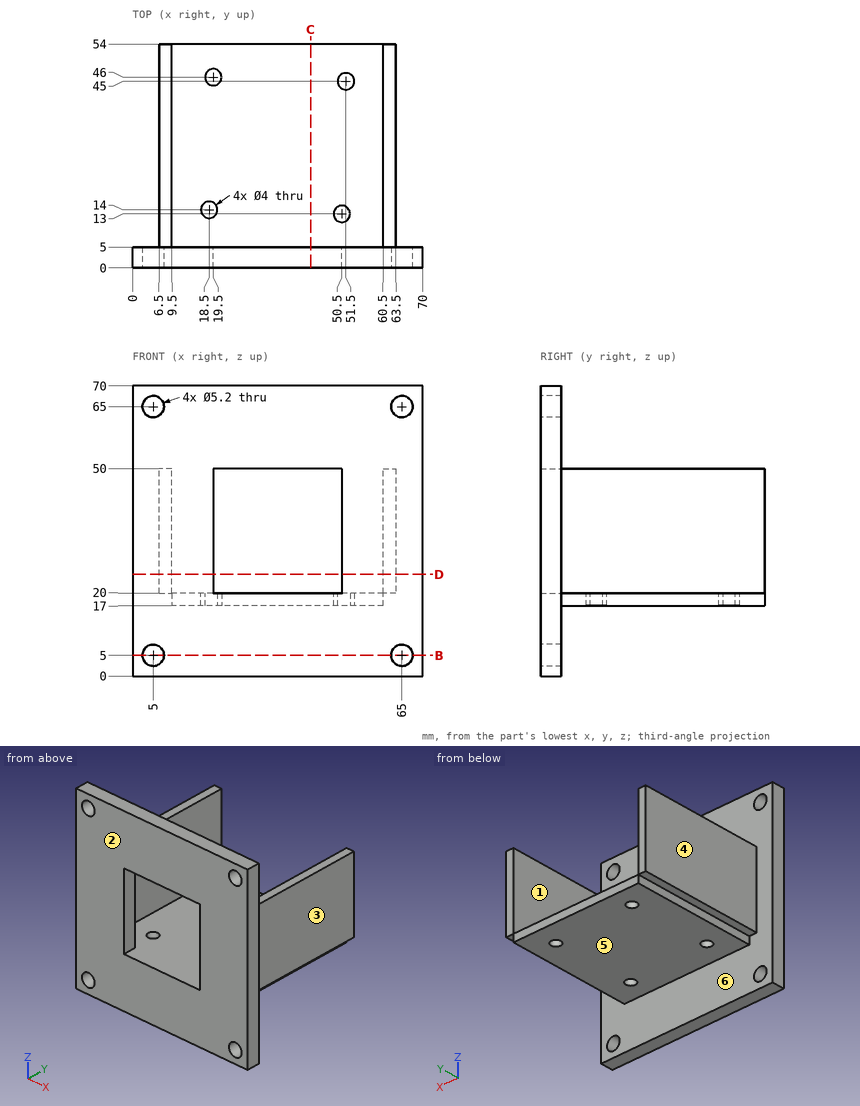
The drawing under review shows one solid part. Ordinate dimensions are in mm from its lowest x, y, z. A direction names the side the tool comes from. Round coordinates to 2 decimals unless told otherwise and drop trailing zeros. Loops run counter-clockwise (first coordinate to the right, second up) from the corner with the lowest first, then second, coordinate; pieces in that order, holes last. Notation, with made-up numbers: (44.25, 80.5) - (84.25, 80.5) arc R13 ccw to (84.25, 102.5) - close; hole circle Ø3 at (30.5, -23.5). An arc over 180 degrees is marked (long way). One line per item, written item: value. Start each with the question number.
1) To check wall thickness, follow L1, parallel to Z at x = 5, y = 1.9; L2, parallel to X at y = 28, z = 22.5; L3, parallel to Z at x = 39, y = 2. State the ranges of each line that lie inside material, in increasing order. Write a range as from..to.
2) Consider section C-C on x = 43. Give the boundary of the cut face in (y, z), then the cut area to 3 significant figures.
3) For the marked faces 1, 2 and 3, list the 3-axis set-ups (+Z, -Z, +X, -X, +Y, -Y) from which the entire face can be reached by the end or side of a thin tool; tool diameter is ignored.
4) Insertion check: pin 1 Ø6 at (x, z) = (58, 18) entering from -Y; pin 2 Ø0.9 at (x, y) = (61.5, 22.5) entering from +Z; pin 3 Ø12 at (y, z) = (41.5, 54) entering from -X; pin 4 Ø2 at (y, z) = (31.5, 28.5) entering from +X. Each pin has a flat end and moves straight along its axis. Give the tip position at first contact, or say it passes through.
5) Consider section D-D on z = 24.5. Give the boundary of the cut face in (x, y).
6) Draft analysis for pull direction X (two halves, no side actions). For the marked faces 4, 5 and 6, state which applies: +X half, -X half, draft (parallel to the pull), parting line (faces both ways), or undercut.
7) Consider section B-B on z = 5. Give the boundary of the cut face in (x, y).
Reported:
1. L1: z = 0..2.4, 7.6..62.4, 67.6..70
1. L2: x = 6.5..9.5, 60.5..63.5
1. L3: z = 0..20, 50..70
2. outline: (0, 0) - (5, 0) - (5, 17) - (54, 17) - (54, 20) - (0, 20) - close; (0, 50) - (5, 50) - (5, 70) - (0, 70) - close
2. area: 347 mm^2
3. face 1: +Z, +Y
3. face 2: +Z, -Z, +X, -X, -Y
3. face 3: +Z, -Z, +X, +Y
4. pin 1: stops at y = 0
4. pin 2: stops at z = 50
4. pin 3: stops at x = 6.5
4. pin 4: stops at x = 63.5
5. outline: (0, 0) - (19.5, 0) - (19.5, 5) - (9.5, 5) - (9.5, 54) - (6.5, 54) - (6.5, 5) - (0, 5) - close; (50.5, 0) - (70, 0) - (70, 5) - (63.5, 5) - (63.5, 54) - (60.5, 54) - (60.5, 5) - (50.5, 5) - close
6. face 4: -X half
6. face 5: draft
6. face 6: undercut
7. outline: (0, 0) - (2.4, 0) - (2.4, 5) - (0, 5) - close; (7.6, 0) - (62.4, 0) - (62.4, 5) - (7.6, 5) - close; (67.6, 0) - (70, 0) - (70, 5) - (67.6, 5) - close
